from build123d import *

# Parameters (mm, degrees)
SKETCH1_W           = 28
SKETCH1_H           = 28
SKETCH1_R           = 1.25
BOSS_EXTRUDE1_DEPTH = 30
SKETCH2_R           = 11
BOSS_EXTRUDE2_DEPTH = 2
SKETCH3_R           = 3
BOSS_EXTRUDE3_DEPTH = 195
FILLET1_R           = 2


with BuildPart() as part:
    # Sketch1 → Boss-Extrude1 (new body)
    with BuildSketch(Plane(origin=(0, 0, 0), x_dir=(1, 0, 0), z_dir=(0, 1, 0))):
        with Locations((14, 14)):
            Rectangle(SKETCH1_W, SKETCH1_H)
        with Locations((2.5, 25.5)):
            Circle(SKETCH1_R, mode=Mode.SUBTRACT)
        with Locations((2.5, 2.5)):
            Circle(SKETCH1_R, mode=Mode.SUBTRACT)
        with Locations((25.5, 2.5)):
            Circle(SKETCH1_R, mode=Mode.SUBTRACT)
        with Locations((25.5, 25.5)):
            Circle(SKETCH1_R, mode=Mode.SUBTRACT)
    extrude(amount=BOSS_EXTRUDE1_DEPTH)

    # Sketch2 → Boss-Extrude2 (add)
    with BuildSketch(Plane(origin=(0, 30, 0), x_dir=(1, 0, 0), z_dir=(0, 1, 0))):
        with Locations((14, 14)):
            Circle(SKETCH2_R)
    extrude(amount=BOSS_EXTRUDE2_DEPTH)

    # Sketch3 → Boss-Extrude3 (add)
    with BuildSketch(Plane(origin=(0, 32, 0), x_dir=(1, 0, 0), z_dir=(0, 1, 0))):
        with Locations((14, 14)):
            Circle(SKETCH3_R)
    extrude(amount=BOSS_EXTRUDE3_DEPTH)

    # Fillet1
    fillet1_edges = [part.edges().sort_by_distance(p)[0] for p in [
        (0, 15, -28),
        (28, 15, -28),
        (28, 15, 0),
        (0, 15, 0),
    ]]
    fillet(fillet1_edges, radius=FILLET1_R)


solid = part.part
Check sheet for the modelled part. Datum: model origin and axes. Units: mm. A direction names the side the tool comes from. Round coordinates to 2 decimals unless told otherwise and drop trailing zeros. Write each loop counter-clockwise with the first axis right and the second up, starting at its lowest first coordinate (ties: lowest second). Pieces come first, ordered by that corner, then holes. Notation, with made-up numbers: (15, 61.5) -> (63, 61.5) arc R13 cw to (63, 75.5) -> close; hole circle Ø3 at (-1, 21). An arc over 180 degrees is marked (long way). Answer as CSV lines item,"result". Start each with the question number.
1) Section check B-B on z = -14. Enter the section's corners in (x, y), and give its area (3 significant figures).
2) Material ranges on line 1 (Z direction, x = 2.5, y = 14.75); line 2 (X direction, y = 8, z = -25.5); line 3 (Y direction, x = 6.25, z = -7.5), recorded low to high. Write a range as from..to.
3) Section check C-C on x = 14. Enter the section's corners in (y, z).
4) Go/stop test with flat-tipped pins: P1, Ø8, axis at x = 8.5, y = 107.5, coming from the +Z side; P2, Ø5, axis at x = 23, z = -17.5, coming from the +Y side; P3, Ø3, axis at y = 65.5, z = -17.5, coming from the +X side; P4, Ø2, axis at x = 25.5, z = -2.5, coming from the +Y side. Record where each tip stops, or that it passes through.
5) Section check D-D on y = 148.5. Enter the section's corners in (x, z).
6) Tool access check on faces 1 (the flat face through (8, 30, -24)), 2 (the flat face through (14, 15, -28)). Record the directions out of +Z, -Z, +X, -X, +Y, -Y that give a thin tool (end or side, any length) a straight path to the whole face; none if there is none.
7) Section check A-A on y = 17. Enter the section's corners in (x, z), and give its area (3 significant figures).
Found:
1,outline,"(0, 0) -> (28, 0) -> (28, 30) -> (25, 30) -> (25, 32) -> (17, 32) -> (17, 227) -> (11, 227) -> (11, 32) -> (3, 32) -> (3, 30) -> (0, 30) -> close"
1,area,"2,050 mm^2"
2,line 1,"z = -28..-26.75, -24.25..-3.75, -1.25..0"
2,line 2,"x = 0..1.25, 3.75..24.25, 26.75..28"
2,line 3,"y = 0..32"
3,outline,"(0, -28) -> (30, -28) -> (30, -25) -> (32, -25) -> (32, -17) -> (227, -17) -> (227, -11) -> (32, -11) -> (32, -3) -> (30, -3) -> (30, 0) -> (0, 0) -> close"
4,P1,"stops at z = -11.4"
4,P2,"stops at y = 32"
4,P3,"stops at x = 16.24"
4,P4,"passes through"
5,outline,"circle Ø6 at (14, -14)"
6,face 1,"+Y"
6,face 2,"-Z, +X, -X, +Y, -Y"
7,outline,"(0, -26) arc R2 ccw to (2, -28) -> (26, -28) arc R2 ccw to (28, -26) -> (28, -2) arc R2 ccw to (26, 0) -> (2, 0) arc R2 ccw to (0, -2) -> close; hole circle Ø2.5 at (2.5, -25.5); hole circle Ø2.5 at (2.5, -2.5); hole circle Ø2.5 at (25.5, -25.5); hole circle Ø2.5 at (25.5, -2.5)"
7,area,"761 mm^2"
